Autodesk Inventor part; units mm, degrees
ref_plane "YZ Plane" through (0, 0, 0) normal (1, 0, 0) x (0, 1, 0)
ref_plane "XZ Plane" through (0, 0, 0) normal (0, 1, 0) x (-1, 0, 0)
ref_plane "XY Plane" through (0, 0, 0) normal (0, 0, 1) x (1, 0, 0)
sketch "Sketch1" plane through (0, 0, 0) normal (0, 1, 0) x (-1, 0, 0)
  line L0 (0, 0) -> (36.5, 0)
  line L1 (36.5, 0) -> (36.5, -66.5)
  line L2 (36.5, -66.5) -> (0, -66.5)
  line L3 (0, -66.5) -> (0, 0)
  line L4 (41.5, 5) -> (-5, 5)
  line L5 (-5, 5) -> (-5, -71.5)
  line L6 (-5, -71.5) -> (41.5, -71.5)
  line L7 (41.5, -71.5) -> (41.5, 5)
  line L8 (18.25, 5) -> (24.25, 5)
  line L9 (18.25, -71.5) -> (24.25, -71.5)
  line L10 (24.25, 5) -> (12.25, 5)
  line L11 (12.25, 5) -> (12.25, 0)
  line L12 (12.25, 0) -> (24.25, 0)
  line L13 (24.25, 0) -> (24.25, 5)
  line L14 (24.25, -71.5) -> (12.25, -71.5)
  line L15 (12.25, -71.5) -> (12.25, -66.5)
  line L16 (12.25, -66.5) -> (24.25, -66.5)
  line L17 (24.25, -66.5) -> (24.25, -71.5)
  dimension "d0" = 36.5
  dimension "d1" = 66.5
  dimension "d2" = 5
  dimension "d3" = 6
  dimension "d4" = 6
  dimension "d5" = 12
  dimension "d6" = 12
extrude "Extrusion1" add sketch "Sketch1" along normal blind 15 contours L3 L2 L15 L6 L5 L4 L11 L0 | L13 L4 L7 L6 L17 L2 L1 L0
sketch "Sketch2" plane through (0, 0, 0) normal (0, -1, 0) x (1, 0, 0)
  line L0 (-12.25, 5) -> (5, 5)
  line L1 (-41.5, -71.5) -> (-41.5, 5)
  line L2 (5, 5) -> (-41.5, 5)
  line L3 (-41.5, 5) -> (-41.5, -71.5)
  line L4 (-41.5, -71.5) -> (5, -71.5)
  line L5 (5, -71.5) -> (5, 5)
  point P0 (0, 0)
extrude "Extrusion2" add sketch "Sketch2" along normal blind 5
sketch "Sketch3" plane through (0, 15, 0) normal (0, 1, 0) x (1, 0, 0)
  line L0 (5, -5) -> (-41.5, -5)
  line L1 (-24.25, -5) -> (-24.25, 0)
  line L2 (-41.5, -5) -> (-24.25, -5)
  line L3 (-24.25, -5) -> (-24.25, 0)
  line L4 (-24.25, 0) -> (-36.5, 0)
  line L5 (-24.25, 0) -> (-36.5, 0)
  line L6 (-36.5, 0) -> (-36.5, 66.5)
  line L7 (-36.5, 0) -> (-36.5, 66.5)
  line L8 (-36.5, 66.5) -> (-24.25, 66.5)
  line L9 (-24.25, 66.5) -> (-24.25, 71.5)
  line L10 (-41.5, 71.5) -> (5, 71.5)
  line L11 (-41.5, -5) -> (-41.5, 71.5)
  line L12 (-41.5, 71.5) -> (-24.25, 71.5)
  line L13 (-41.5, 71.5) -> (-41.5, -5)
  line L14 (-12.25, 0) -> (-12.25, -5)
  line L15 (-12.25, -5) -> (5, -5)
  line L16 (5, -5) -> (5, 71.5)
  line L17 (5, -5) -> (5, 71.5)
  line L18 (5, 71.5) -> (-12.25, 71.5)
  line L19 (-12.25, 71.5) -> (-12.25, 66.5)
  line L20 (-12.25, 66.5) -> (-12.25, 71.5)
  line L21 (0, 0) -> (-12.25, 0)
  line L22 (-12.25, -5) -> (-12.25, 0)
  line L23 (-12.25, 0) -> (0, 0)
  line L24 (0, 66.5) -> (0, 0)
  line L25 (0, 0) -> (0, 66.5)
  line L26 (-12.25, 66.5) -> (0, 66.5)
  line L27 (0, 66.5) -> (-12.25, 66.5)
properties part number "voltage buckboost cover"
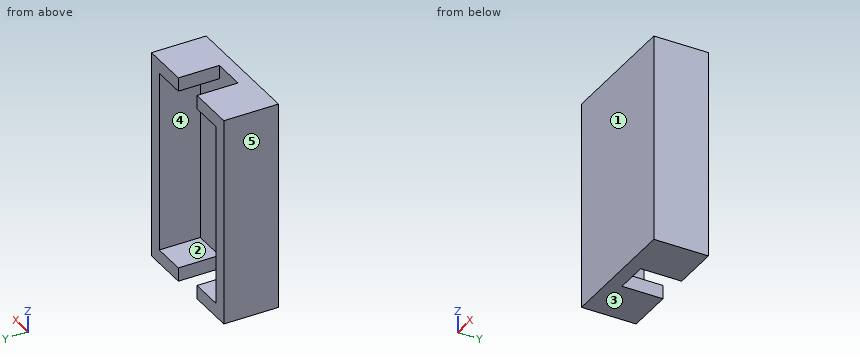
Could you check a few things on this model? Use its own coordinates, in mm. Face numbers are marked on the shaded views. A direction names the side the tool comes from. Give positions to 0.01 mm unless a question says otherwise; leave off trailing zeros. Order: outer loops, then holes, each group sorted by start corner. A loop starts at its lowest first (then second) coordinate and runs counter-clockwise, first axis right, second up. Notation, with made-up numbers: (-40, 61.5) -> (-8, 61.5) arc R6 cw to (-8, 71.5) -> close; hole circle Ø4 at (17, 68). An arc over 180 degrees is marked (long way). Answer in a Markdown table with one row per item. Add a question column.
Item 1: Please list where these lines run through material, in increasing order: probe 1 along X at (y, z) = (3.5, -39); probe 2 along Z at (x, y) = (-8, 2.5); probe 3 along Y at (x, z) = (-28, -16).
Item 2: I'm going to push a flat-ended pin straight in: P1, Ø8, axis at x = -21.5, y = 11.5, coming from the +Z side. Where does the tip first touch, or does it pass through?
Item 3: Imagine slicing it at B-B (z = -23.5). List the corners of the cut face in (x, y) for me, and give its area (4 significant figures).
Item 4: Imagine slicing it at C-C (x = -34.5). List the corners of the cut face in (y, z) for me.
Item 5: We'd pull the mould along Z, two halves only. Please class the marked faces 1, 2 and 3: pulls with the +Z half, pulls with the -Z half, needs draft (parallel to the pull), parting line crosses it, or undercut.
Item 6: For the marked faces 4 and 5, which set-ups out of +Z, -Z, +X, -X, +Y, -Y let a thin tool reach every point of the face, with its end or its side?
Item 7: Imagine slicing it at A-A (y = 12). List the corners of the cut face in (x, z) for me, and give its area (3 significant figures).
Item 8: Imagine slicing it at D-D (x = -21.5). List the corners of the cut face in (y, z) for me, and give its area (4 significant figures).
Result:
| question | item | result |
|---|---|---|
| 1 | probe 1 | -41.5 to -36.5, 0 to 5 |
| 1 | probe 2 | -71.5 to -66.5, 0 to 5 |
| 1 | probe 3 | -5 to 0 |
| 2 | P1 | z = 5 |
| 3 | outline | (-41.5, -5) -> (5, -5) -> (5, 15) -> (0, 15) -> (0, 0) -> (-36.5, 0) -> (-36.5, 15) -> (-41.5, 15) -> close |
| 3 | area | 382.5 mm2 |
| 4 | outline | (-5, -71.5) -> (15, -71.5) -> (15, -66.5) -> (0, -66.5) -> (0, 0) -> (15, 0) -> (15, 5) -> (-5, 5) -> close |
| 5 | face 1 | needs draft |
| 5 | face 2 | undercut |
| 5 | face 3 | pulls with the -Z half |
| 6 | face 4 | +Y |
| 6 | face 5 | +Z, -Z, -X, +Y, -Y |
| 7 | outline | (-41.5, -71.5) -> (-24.25, -71.5) -> (-24.25, -66.5) -> (-36.5, -66.5) -> (-36.5, 0) -> (-24.25, 0) -> (-24.25, 5) -> (-41.5, 5) -> close; (-12.25, -71.5) -> (5, -71.5) -> (5, 5) -> (-12.25, 5) -> (-12.25, 0) -> (0, 0) -> (0, -66.5) -> (-12.25, -66.5) -> close |
| 7 | area | 1,010 mm2 |
| 8 | outline | (-5, -71.5) -> (0, -71.5) -> (0, 5) -> (-5, 5) -> close |
| 8 | area | 382.5 mm2 |
